For this review, take the finished solid that the model builds, in its own axes (mm). Face numbers are marked on the shaded views. A direction names the side the tool comes from. Round coordinates to 2 decimals unless told otherwise and drop trailing zeros. Order: outer loops, then holes, each group sorted by start corner. A loop starts at its lowest first (then second) coordinate and runs counter-clockwise, first axis right, second up. Notation, with made-up numbers: M 63,89 L 104,89 A6 cw 104,100 Z; hole C 46,16 d6. An arc over 180 degrees is marked long. Use a Markdown table: item, result.
from build123d import *

# Parameters (mm, degrees)
SKETCH1_R           = 5.4
BOSS_EXTRUDE1_DEPTH = 12.7
SKETCH3_R           = 1.5
CUT_EXTRUDE2_DEPTH  = 12.7
SKETCH5_R           = 2.25
CUT_EXTRUDE3_DEPTH  = 3.5
SKETCH4_R           = 3.2
CUT_EXTRUDE4_DEPTH  = 9.2


with BuildPart() as part:
    # Sketch1 → Boss-Extrude1 (new body)
    with BuildSketch(Plane.XY):
        Circle(SKETCH1_R)
    extrude(amount=BOSS_EXTRUDE1_DEPTH)

    # Sketch3 → Cut-Extrude2 (cut)
    with BuildSketch(Plane(origin=(0, 5.4, 0), x_dir=(1, 0, 0), z_dir=(0, 1, 0))):
        with Locations(Location((0, -8.486582987, 0), (0, 0, 270))):
            Circle(SKETCH3_R)
    extrude(amount=-CUT_EXTRUDE2_DEPTH, mode=Mode.SUBTRACT)

    # Sketch5 → Cut-Extrude3 (cut)
    with BuildSketch(Plane(origin=(0, 0, 0), x_dir=(-1, 0, 0), z_dir=(0, 0, -1))):
        Circle(SKETCH5_R)
    extrude(amount=-CUT_EXTRUDE3_DEPTH, mode=Mode.SUBTRACT)

    # Sketch4 → Cut-Extrude4 (cut)
    with BuildSketch(Plane.XY.offset(12.7)):
        Circle(SKETCH4_R)
    extrude(amount=-CUT_EXTRUDE4_DEPTH, mode=Mode.SUBTRACT)


solid = part.part
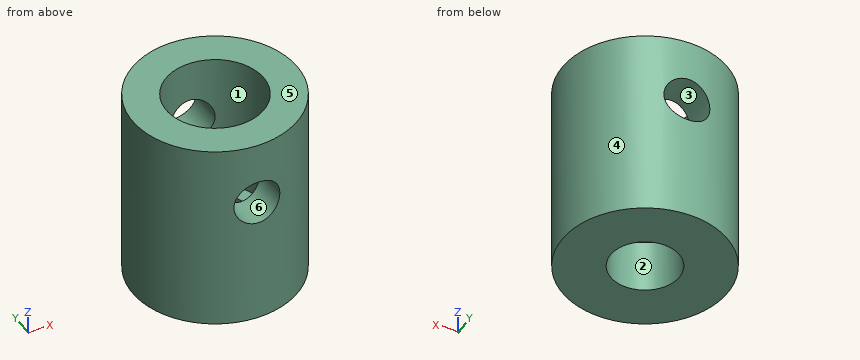
Q1. Add section A-A (x = 0). Write out the cut boundary in (y, z), then the cut area to 3 significant figures.
Determined:
| item | result |
|---|---|
| outline | M -5.4,0 L -2.25,0 L -2.25,3.5 L -3.2,3.5 L -3.2,6.99 L -5.4,6.99 Z; M -5.4,9.99 L -3.2,9.99 L -3.2,12.7 L -5.4,12.7 Z; M 2.25,0 L 5.4,0 L 5.4,6.99 L 3.2,6.99 L 3.2,3.5 L 2.25,3.5 Z; M 3.2,9.99 L 5.4,9.99 L 5.4,12.7 L 3.2,12.7 Z |
| area | 49.3 mm^2 |
Q2. Wall thickness on line 1 along Y through (x, z) = (0, 2.25); line 2 along Z through (x, y) = (0, 4.8); line 3 along Z through (x, y) = (-1.5, -2.5): over which ranges is each line inside the solid? List them lowest first. Write a range as [from, to].
Determined:
| item | result |
|---|---|
| line 1 | y = [-5.4, -2.25], [2.25, 5.4] |
| line 2 | z = [0, 6.99], [9.99, 12.7] |
| line 3 | z = [0, 3.5] |
Q3. Clearance check with flat-ended pins moving along their axes: pin 1 (3 mm diameter, centred on x = 2.5, y = 0.5, fed in from +Z); pin 2 (2.5 mm diameter, centred on x = 0, z = 8.49, fed in from -Y); pin 3 (2 mm diameter, centred on x = -1.5, z = 8.5, fed in from -Y); pin 4 (5 mm diameter, centred on x = 0, y = 0, fed in from +Z). State where each tip first meets the part, or that it passes through.
Determined:
| item | result |
|---|---|
| pin 1 | stops at z = 12.7 |
| pin 2 | passes through |
| pin 3 | stops at y = -5.27 |
| pin 4 | stops at z = 3.5 |
Q4. Draft analysis for pull direction X (two halves, no side actions). For the marked faces 3, 4, 5 and 6, state which applies: pulls with the +X half, pulls with the -X half, needs draft (parallel to the pull), parting line crosses it, or undercut.
Determined:
| item | result |
|---|---|
| face 3 | undercut |
| face 4 | parting line crosses it |
| face 5 | needs draft |
| face 6 | undercut |
Q5. Add section C-C (z = 8). Write out the cut boundary in (x, y), then the cut area to 3 significant figures.
Determined:
| item | result |
|---|---|
| outline | M -1.42,-5.21 L -1.42,-2.87 A3.2 cw -1.42,2.87 L -1.42,5.21 A5.4 ccw Z; M 1.42,-5.21 A5.4 ccw 1.42,5.21 L 1.42,2.87 A3.2 cw 1.42,-2.87 Z |
| area | 46.7 mm^2 |
Q6. Add section B-B (y = 0). Write out the cut boundary in (x, z), then the cut area to 3 significant figures.
Determined:
| item | result |
|---|---|
| outline | M -5.4,0 L -2.25,0 L -2.25,3.5 L -3.2,3.5 L -3.2,12.7 L -5.4,12.7 Z; M 2.25,0 L 5.4,0 L 5.4,12.7 L 3.2,12.7 L 3.2,3.5 L 2.25,3.5 Z |
| area | 62.5 mm^2 |
Q7. Machinability: for the marked faces 1 and 2, which of the approach directions +Z, -Z, +X, -X, +Y, -Y give a long, thin tool a straight path to every point of the face, cutting with its end or side? Answer none if there is none.
Determined:
| item | result |
|---|---|
| face 1 | +Z |
| face 2 | +Z, -Z |
Q8. Add section D-D (x = -2). Write out the cut boundary in (y, z).
Determined:
| item | result |
|---|---|
| outline | M -5.02,0 L -1.03,0 L -1.03,3.5 L -2.5,3.5 L -2.5,12.7 L -5.02,12.7 Z; M 1.03,0 L 5.02,0 L 5.02,12.7 L 2.5,12.7 L 2.5,3.5 L 1.03,3.5 Z |
